Study the drawing (mm; zero at the part's minimum x, y, z) and answer. Coordinates: 2 decimals unless noted, no trailing zeros. Write each loop counter-clockwise with the first axis right and the second up, starting at its lowest first coordinate (ties: lowest second). Pieces come first, ordered by that corner, then holes. Notation, with made-up numbers: (51, 59.5) - (87, 59.5) arc R20 cw to (87, 66.5) - close; hole circle Ø3 at (-35.5, 85.5). An arc over 180 degrees is marked (long way). One line per item, written item: value.
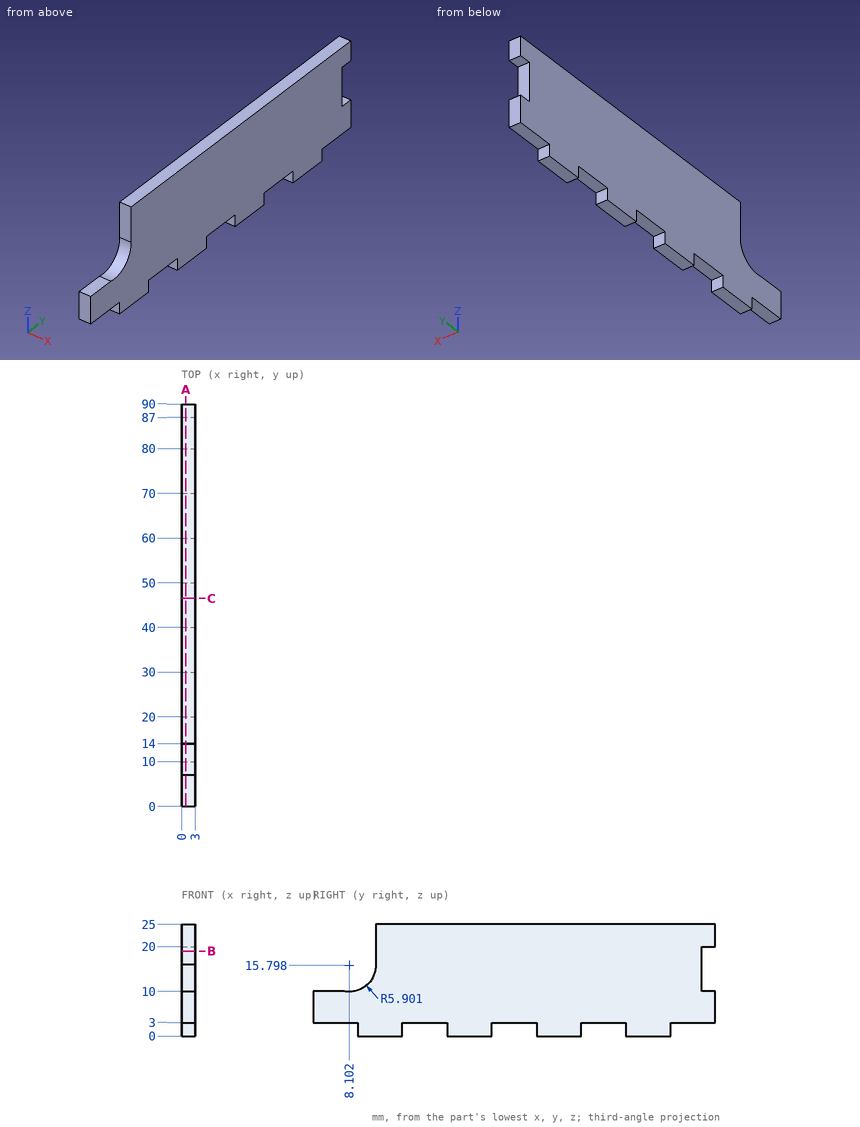
Item 1: Section A-A, the plane x = 0.95 is taken. Determine the outline of the cut face in (y, z).
Evaluation:
outline: (0, 3) - (10, 3) - (10, 0) - (20, 0) - (20, 3) - (30, 3) - (30, 0) - (40, 0) - (40, 3) - (50, 3) - (50, 0) - (60, 0) - (60, 3) - (70, 3) - (70, 0) - (80, 0) - (80, 3) - (90, 3) - (90, 10) - (87, 10) - (87, 20) - (90, 20) - (90, 25) - (14, 25) - (14, 16) arc R5.9 cw to (7, 10) - (0, 10) - close
Item 2: Section C-C, the plane y = 46.5 is taken. Determine the outline of the cut face in (x, z).
Evaluation:
outline: (0, 3) - (3, 3) - (3, 25) - (0, 25) - close
Item 3: Given pin 1 (0.9 mm diameter, centred on x = 2, y = 6, fed in from -Z); pin 2 (0.9 mm diameter, centred on x = 2, z = 2, fed in from -Y); pin 3 (0.9 mm diameter, centred on x = 2, z = 1, fed in from +Y), each flat-ended and moving along its own axis, determine where each tip first touches the part or whether it passes through.
Evaluation:
pin 1: stops at z = 3
pin 2: stops at y = 10
pin 3: stops at y = 80
Item 4: Section B-B, the plane z = 19 is taken. Determine the outline of the cut face in (x, y).
Evaluation:
outline: (0, 14) - (3, 14) - (3, 87) - (0, 87) - close
Item 5: Consider probe 1 along Z at (x, y) = (0.8, 68); probe 2 along Y at (x, z) = (0.2, 19.25); probe 3 along Y at (x, z) = (2.85, 20.5). Determine where each line is inside the solid, lowest interval first.
Evaluation:
probe 1: z = 3 to 25
probe 2: y = 14 to 87
probe 3: y = 14 to 90
